Read the model definition and answer for the solid it produces. Units are mm, in the model's axes. Face numbers are marked on the shaded views. A direction names the side the tool comes from. Round coordinates to 2 decimals unless told otherwise and drop trailing zeros. Write each loop counter-clockwise with the first axis right and the second up, starting at its lowest first coordinate (ties: lowest second). Pieces come first, ordered by that corner, then holes.
from build123d import *

# Parameters (mm, degrees)
F1_DEPTH = 34.08
F2_R     = 4.035
F3_DEPTH = 7.131
F4_R     = 1
F2_W     = 9.985
F2_H     = 4.77
F5_DEPTH = 27.1
F6_START = -3.4
F6_DEPTH = 23.7


with BuildPart() as f1:
    # F0 (on Top) → F1 (new body)
    with BuildSketch(Plane.XY):
        Polygon((27.1, 37.69), (23.7, 37.69), (23.7, 2.76), (19.97, 2.76), (19.97, -34.99), (23.7, -34.99), (23.7, 0), (27.1, 0), align=None)
    extrude(amount=F1_DEPTH)

    # F2 (on face) → F3 (cut, through all)
    with BuildSketch(Plane.YZ.offset(27.1)):
        with Locations((24.595, 17.04)):
            Circle(F2_R)
        with BuildLine():
            Line((37.69, 34.08), (24.595, 34.08))
            ThreePointArc((24.595, 34.08), (31.8257980304, 32.4697491828), (37.69, 27.9433286202))
            Line((37.69, 27.9433286202), (37.69, 34.08))
        make_face()
        with BuildLine():
            Line((37.69, 0), (37.69, 6.1366713798))
            ThreePointArc((37.69, 6.1366713798), (31.8257980304, 1.6102508172), (24.595, 0))
            Line((24.595, 0), (37.69, 0))
        make_face()
    extrude(amount=-F3_DEPTH, mode=Mode.SUBTRACT)

    # F4
    f4_edges = [f1.edges().sort_by_distance(p)[0] for p in [
        (25.4, 37.69, 6.136671),
        (25.4, 37.69, 27.943329),
        (19.97, 2.76, 17.04),
    ]]
    fillet(f4_edges, radius=F4_R)

    # F2 (on face) → F5 (join, through all)
    with BuildSketch(Plane.YZ.offset(27.1)):
        with Locations((4.9925, 2.385)):
            Rectangle(F2_W, F2_H)
    extrude(amount=-F5_DEPTH)

    # F2 (on face) → F6 (join)
    with BuildSketch(Plane.YZ.offset(27.1).offset(F6_START)):
        with Locations((-4.9925, 2.385)):
            Rectangle(F2_W, F2_H)
    extrude(amount=-F6_DEPTH)


solid = f1.part
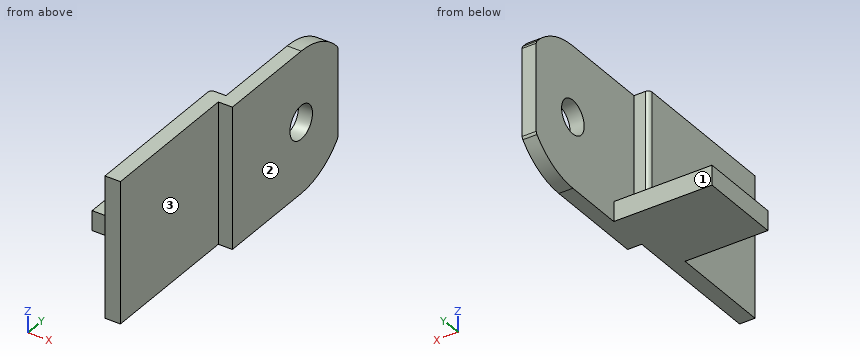
Q1. Section B-B (y = 25.5) is taken. Determine the outline of the cut face in (x, z), then the cut area to 3 significant figures.
Verdict:
outline: (23.7, 0.02) - (27.1, 0.02) - (27.1, 13.11) - (23.7, 13.11) - close; (23.7, 20.97) - (27.1, 20.97) - (27.1, 34.06) - (23.7, 34.06) - close
area: 89.0 mm2
Q2. Section A-A (z = 17.04) is taken. Determine the outline of the cut face in (x, y), then the cut area to 3 significant figures.
Verdict:
outline: (19.97, -34.99) - (23.7, -34.99) - (23.7, 0) - (27.1, 0) - (27.1, 20.56) - (23.7, 20.56) - (23.7, 2.76) - (20.97, 2.76) arc R1 ccw to (19.97, 1.76) - close; (23.7, 28.63) - (27.1, 28.63) - (27.1, 37.69) - (23.7, 37.69) - close
area: 241 mm2
Q3. Straight lines are drawn through the part: probe 1 along X at (y, z) = (-25.5, 15); probe 2 along X at (y, z) = (18.5, 8.5); probe 3 along Y at (x, z) = (22.5, 9). For each, find the intervals that lie inside material, in ascending order.
Verdict:
probe 1: x = 19.97 to 23.7
probe 2: x = 23.7 to 27.1
probe 3: y = -34.99 to 2.76
Q4. Section D-D (y = -8) is taken. Determine the outline of the cut face in (x, z).
Verdict:
outline: (0, 0) - (23.7, 0) - (23.7, 34.08) - (19.97, 34.08) - (19.97, 4.77) - (0, 4.77) - close
Q5. Flat-ended cylindrical pins translate along their axes: pin 1 Ø7.5 at (y, z) = (24.595, 17.04) entering from +X; pin 2 Ø6 at (y, z) = (-11.5, 25.5) entering from +X; pin 3 Ø10 at (x, y) = (13.5, 4) entering from +Z; pin 4 Ø3.5 at (x, z) = (26, 11.5) entering from -Y. Find the tip coordinate at first contact, or state that the pin passes through.
Verdict:
pin 1: passes through
pin 2: stops at x = 23.7
pin 3: stops at z = 4.77
pin 4: stops at y = 0
Q6. Section C-C (x = 22.25) is taken. Determine the outline of the cut face in (y, z) (3 decimals).
Verdict:
outline: (-34.99, 0) - (9.985, 0) - (9.985, 4.77) - (2.76, 4.77) - (2.76, 34.08) - (-34.99, 34.08) - close
Q7. Which of the six approach directions +Z, -Z, +X, -X, +Y, -Y give full straight-line access (tool end or side, diameter ignored) to the marked faces 1, 2 and 3?
Verdict:
face 1: +Z, -Z, -X, +Y
face 2: +Z, -Z, +X, +Y, -Y
face 3: +Z, -Z, +X, -Y
